Read the model definition and answer for the solid it produces. Units are mm, in the model's axes. Give positions to 0.01 mm unless a question says otherwise; leave off trailing zeros. Order: outer loops, then holes, each group sorted by start corner. A loop starts at its lowest first (then second) coordinate and runs counter-clockwise, first axis right, second up. Notation, with made-up numbers: (87.5, 68.5) - (137.5, 68.5) arc R19 ccw to (137.5, 74.5) - close; hole circle Ø11 at (0.25, 71.25). An arc over 180 degrees is marked (long way). Return JSON: item names as keys, results as strings.
```python
from build123d import *

# Parameters (mm, degrees)
SKETCH1_R           = 0.5
BOSS_EXTRUDE1_DEPTH = 0.8


with BuildPart() as part:
    # Sketch1 → Boss-Extrude1 (new body)
    with BuildSketch(Plane.XY):
        with BuildLine():
            Line((4.25, 0), (4.25, -11))
            Line((4.25, -11), (-4.25, -11))
            Line((-4.25, -11), (-4.25, 0))
            ThreePointArc((-4.25, 0), (0, 4.25), (4.25, 0))
        make_face()
        with Locations((0, -2.3)):
            Circle(SKETCH1_R, mode=Mode.SUBTRACT)
        with Locations((-1.991858429, 1.15)):
            Circle(SKETCH1_R, mode=Mode.SUBTRACT)
        with Locations((1.991858429, 1.15)):
            Circle(SKETCH1_R, mode=Mode.SUBTRACT)
    extrude(amount=BOSS_EXTRUDE1_DEPTH)


solid = part.part
```
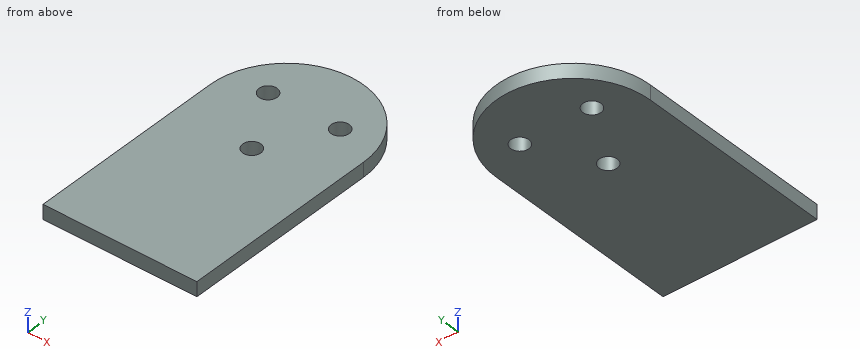
Q1. A cutting plane is placed at A-A (y = -2). Write down the section's boundary in (x, z).
Values:
{"outline": "(-4.25, 0) - (-0.4, 0) - (-0.4, 0.8) - (-4.25, 0.8) - close; (0.4, 0) - (4.25, 0) - (4.25, 0.8) - (0.4, 0.8) - close"}
Q2. A cutting plane is placed at B-B (x = 0). Write down the section's boundary in (y, z), and give its area (3 significant figures).
Values:
{"outline": "(-11, 0) - (-2.8, 0) - (-2.8, 0.8) - (-11, 0.8) - close; (-1.8, 0) - (4.25, 0) - (4.25, 0.8) - (-1.8, 0.8) - close", "area": "11.4 mm²"}
Q3. A cutting plane is placed at D-D (y = 3.25). Write down the section's boundary in (x, z).
Values:
{"outline": "(-2.74, 0) - (2.74, 0) - (2.74, 0.8) - (-2.74, 0.8) - close"}
Q4. A cutting plane is placed at C-C (z = 0.45). Write down the section's boundary in (x, y).
Values:
{"outline": "(-4.25, -11) - (4.25, -11) - (4.25, 0) arc R4.25 ccw to (-4.25, 0) - close; hole circle Ø1 at (-1.99, 1.15); hole circle Ø1 at (0, -2.3); hole circle Ø1 at (1.99, 1.15)"}
Q5. Consider L1, parallel to X at y = 1.5, z = 0.7; L2, parallel to Y at x = -3.5, z = 0.25; L3, parallel to Y at x = 2.75, z = 0.4. Determine where each line is inside the solid, lowest interval first.
Values:
{"L1": "x = -3.98 to -2.35, -1.63 to 1.63, 2.35 to 3.98", "L2": "y = -11 to 2.41", "L3": "y = -11 to 3.24"}
